Model file for the job. Use its own axes, mm. Face numbers are marked on the shaded views. A direction names the side the tool comes from. Round coordinates to 2 decimals unless told otherwise and drop trailing zeros. Loops run counter-clockwise (first coordinate to the right, second up) from the corner with the lowest first, then second, coordinate; pieces in that order, holes last. Notation, with made-up numbers: (70.5, -39) - (118.5, -39) arc R37 cw to (118.5, -1) - close; hole circle Ø9 at (-27, 5). An arc over 180 degrees is marked (long way). Answer as a JSON object with one key per item and string values.
from build123d import *

# Parameters (mm, degrees)
F1_DEPTH = 60
F3_DEPTH = 20
F5_DEPTH = 20
F6_R     = 8
F7_DEPTH = 80


with BuildPart() as f1:
    # F0 (on Front) → F1 (new body)
    with BuildSketch(Plane.XZ):
        with BuildLine():
            Line((-71.441528, 48.114919), (-81.441528, 48.114919))
            Line((-81.441528, 48.114919), (-81.441528, 8.114919))
            Line((-81.441528, 8.114919), (-121.441528, 8.114919))
            Line((-121.441528, 8.114919), (-121.441528, -11.885081))
            Line((-121.441528, -11.885081), (38.558472, -11.885081))
            Line((38.558472, -11.885081), (38.558472, 8.114919))
            Line((38.558472, 8.114919), (-1.441528, 8.114919))
            Line((-1.441528, 8.114919), (-1.441528, 48.114919))
            Line((-1.441528, 48.114919), (-11.441528, 48.114919))
            ThreePointArc((-11.441528, 48.114919), (-41.441528, 18.114919), (-71.441528, 48.114919))
        make_face()
    extrude(amount=F1_DEPTH)

    # F2 (on face) → F3 (cut)
    with BuildSketch(Plane.XY.offset(8.114919)):
        with BuildLine():
            Line((29.558472, -45), (29.558472, -15))
            ThreePointArc((29.558472, -15), (23.558472, -9), (17.558472, -15))
            Line((17.558472, -15), (17.558472, -45))
            ThreePointArc((17.558472, -45), (23.558472, -51), (29.558472, -45))
        make_face()
    extrude(amount=-F3_DEPTH, mode=Mode.SUBTRACT)

    # F4 (on face) → F5 (cut)
    with BuildSketch(Plane.XY.offset(8.114919)):
        with BuildLine():
            Line((-112.441528, -15), (-112.441528, -45))
            ThreePointArc((-112.441528, -45), (-106.441528, -51), (-100.441528, -45))
            Line((-100.441528, -45), (-100.441528, -15))
            ThreePointArc((-100.441528, -15), (-106.441528, -9), (-112.441528, -15))
        make_face()
    extrude(amount=-F5_DEPTH, mode=Mode.SUBTRACT)

    # F6 (on face) → F7 (cut)
    with BuildSketch(Plane.YZ.offset(-1.441528)):
        with Locations((-30, 33.114919)):
            Circle(F6_R)
    extrude(amount=-F7_DEPTH, mode=Mode.SUBTRACT)

    # F8: F1 across face


with BuildPart() as f1_1:
    add(f1.part)
    add(f1.part.mirror(Plane(origin=(-41.441528, -60, 6.801582), x_dir=(1, 0, 0), z_dir=(0, -1, 0))))


solid = f1_1.part
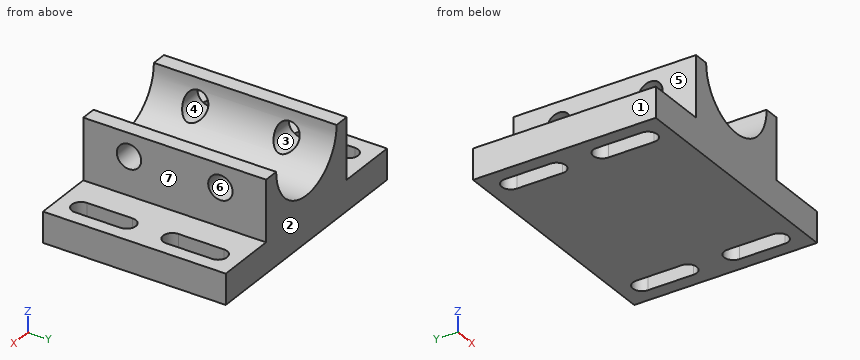
1) Slice it at A-A on y = -90. List the corners of the cut face in (x, z), then the cut area to 3 significant figures.
Values follow:
{"outline": "(-121.44, -11.89) - (-112.44, -11.89) - (-112.44, 8.11) - (-121.44, 8.11) - close; (-100.44, -11.89) - (17.56, -11.89) - (17.56, 8.11) - (-1.44, 8.11) - (-1.44, 25.11) - (-22.18, 25.11) arc R30 cw to (-60.7, 25.11) - (-81.44, 25.11) - (-81.44, 8.11) - (-100.44, 8.11) - close; (-81.44, 41.11) - (-70.61, 41.11) arc R30 cw to (-71.44, 48.11) - (-81.44, 48.11) - close; (-12.27, 41.11) - (-1.44, 41.11) - (-1.44, 48.11) - (-11.44, 48.11) arc R30 cw to start; (29.56, -11.89) - (38.56, -11.89) - (38.56, 8.11) - (29.56, 8.11) - close", "area": "4,040 mm²"}
2) Slice it at B-B on z = -8. List the corners of the cut face in (x, y).
Values follow:
{"outline": "(-121.44, -120) - (38.56, -120) - (38.56, 0) - (-121.44, 0) - close; hole (-112.44, -105) arc R6 ccw to (-100.44, -105) - (-100.44, -75) arc R6 ccw to (-112.44, -75) - close; hole (-112.44, -45) arc R6 ccw to (-100.44, -45) - (-100.44, -15) arc R6 ccw to (-112.44, -15) - close; hole (17.56, -105) arc R6 ccw to (29.56, -105) - (29.56, -75) arc R6 ccw to (17.56, -75) - close; hole (17.56, -45) arc R6 ccw to (29.56, -45) - (29.56, -15) arc R6 ccw to (17.56, -15) - close"}
3) Probe probe 1 along X at (y, z) = (-96, 3); probe 2 along Z at (x, y) = (-9, -29.5); probe 3 along X at (y, z) = (-12, 5). List the from-to ranges inside material, lowest first.
Values follow:
{"probe 1": "-121.44 to -112.44, -100.44 to 17.56, 29.56 to 38.56", "probe 2": "-11.89 to 25.13, 41.1 to 48.11", "probe 3": "-121.44 to -111.64, -101.25 to 18.36, 28.75 to 38.56"}
4) Slice it at D-D on x = -76. List the corners of the cut face in (y, z), then the cut area to 3 significant figures.
Values follow:
{"outline": "(-120, -11.89) - (0, -11.89) - (0, 48.11) - (-120, 48.11) - close; hole circle Ø16 at (-90, 33.11); hole circle Ø16 at (-30, 33.11)", "area": "6,800 mm²"}
5) Drop flat-ended pins along their axis: P1, Ø12, axis at y = -49.5, z = 37.5, coming from the +X side; P2, Ø4, axis at x = -94.5, y = -86, coming from the +Z side; P3, Ø9.5, axis at y = -30, z = 33.11, coming from the +X side. Give the stop position or say it passes through.
Values follow:
{"P1": "x = -1.44", "P2": "z = 8.11", "P3": "through"}
6) Two-plate mould, pull along Y, no slides. Class the marked faces 1, 2, 3 and 4: pulls with the +Y half, pulls with the -Y half, needs draft (parallel to the pull), parting line crosses it, or undercut.
Values follow:
{"face 1": "needs draft", "face 2": "pulls with the +Y half", "face 3": "undercut", "face 4": "undercut"}
7) Tool access for the marked faces 5, 6 and 7: list every direction of +Z, -Z, +X, -X, +Y, -Y with a clear straight run to the whole face (end or side of a thin tool).
Values follow:
{"face 5": "+Z, -X, +Y, -Y", "face 6": "+X, -X", "face 7": "+Z, +X, +Y, -Y"}
8) Slice it at C-C on y = -108. List the corners of the cut face in (x, z), then the cut area to 3 significant figures.
Values follow:
{"outline": "(-121.44, -11.89) - (-111.64, -11.89) - (-111.64, 8.11) - (-121.44, 8.11) - close; (-101.25, -11.89) - (18.36, -11.89) - (18.36, 8.11) - (-1.44, 8.11) - (-1.44, 48.11) - (-11.44, 48.11) arc R30 cw to (-71.44, 48.11) - (-81.44, 48.11) - (-81.44, 8.11) - (-101.25, 8.11) - close; (28.75, -11.89) - (38.56, -11.89) - (38.56, 8.11) - (28.75, 8.11) - close", "area": "4,570 mm²"}
